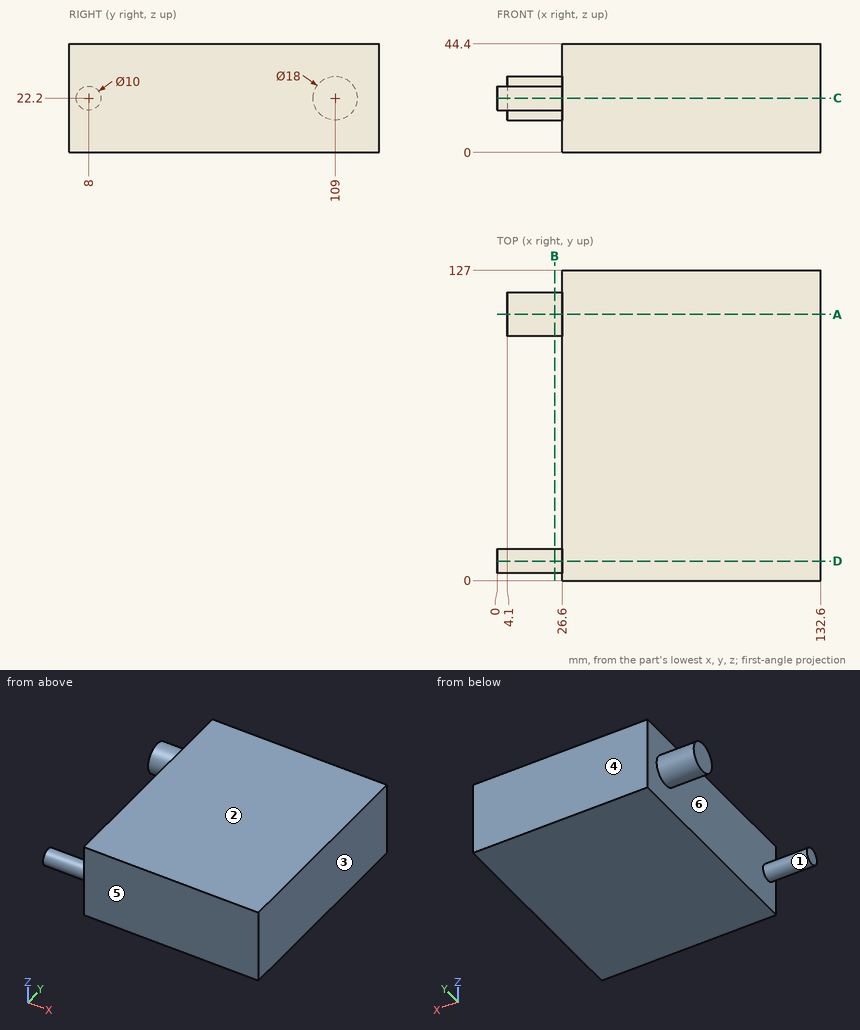
For this review, use the dimensioned drawing (mm, ordinates from the lowest corner) and the shaded views. A direction names the side the tool comes from. Coordinates: 2 decimals unless noted, no trailing zeros. Order: outer loops, then holes, each group sorted by start corner. A loop starts at its lowest first (then second) coordinate and runs counter-clockwise, first axis right, second up. Notation, with made-up numbers: (22, 78) - (44, 78) arc R26 cw to (44, 108) - close; hole circle Ø1 at (-32, 0.5). An arc over 180 degrees is marked (long way). Answer as a JSON object with one key per item and string values. Group by question number.
1. We need section A-A on y = 109. State the section outline as (x, z) points, then the cut area to 3 significant figures.
2. For the marked faces 1 and 2, list the 3-axis set-ups (+Z, -Z, +X, -X, +Y, -Y) from which the entire face can be reached by the end or side of a thin tool; tool diameter is ignored.
3. Clearance check with flat-ended pins moving along their axes: P1, Ø8, axis at y = 102.5, z = 23, coming from the -X side; P2, Ø2, axis at y = 68, z = 33.5, coming from the -X side. State where each tip first meets the part, or that it passes through.
4. The part is to be moulded in two halves that separate along Y. For the marked faces 3, 4, 5 and 6, say which applies: pulls with the +Y half, pulls with the -Y half, needs draft (parallel to the pull), parting line crosses it, or undercut.
5. For probe 1 along X at (y, z) = (95, 10.5), list the stretches that pass through material, from the lowest coordinate up.
6. We need section D-D on y = 8. State the section outline as (x, z) points.
7. We need section B-B on x = 23.5. State the section outline as (y, z) points.
8. We need section C-C on z = 22.2. State the section outline as (x, y) points, then the cut area to 3 significant figures.
Final values:
{
 "1": {"outline": "(4.1, 13.2) - (26.6, 13.2) - (26.6, 0) - (132.6, 0) - (132.6, 44.4) - (26.6, 44.4) - (26.6, 31.2) - (4.1, 31.2) - close", "area": "5,110 mm²"},
 "2": {"face 1": "-X", "face 2": "+Z, +X, -X, +Y, -Y"},
 "3": {"P1": "x = 4.1", "P2": "x = 26.6"},
 "4": {"face 3": "needs draft", "face 4": "pulls with the +Y half", "face 5": "pulls with the -Y half", "face 6": "undercut"},
 "5": {"probe 1": "26.6 to 132.6"},
 "6": {"outline": "(0, 17.2) - (26.6, 17.2) - (26.6, 0) - (132.6, 0) - (132.6, 44.4) - (26.6, 44.4) - (26.6, 27.2) - (0, 27.2) - close"},
 "7": {"outline": "circle Ø10 at (8, 22.2); circle Ø18 at (109, 22.2)"},
 "8": {"outline": "(0, 3) - (26.6, 3) - (26.6, 0) - (132.6, 0) - (132.6, 127) - (26.6, 127) - (26.6, 118) - (4.1, 118) - (4.1, 100) - (26.6, 100) - (26.6, 13) - (0, 13) - close", "area": "14,100 mm²"}
}
